Verification items for this drawing (mm, ordinates from the low corner). Round coordinates to 2 decimals unless told otherwise and drop trailing zeros. Loops run counter-clockwise (first coordinate to the right, second up) from the corner with the lowest first, then second, coordinate; pieces in that order, holes last. Notation, with made-up numbers: (-11, -9) - (25, -9) arc R7 cw to (25, 4) - close; hole circle Ø6 at (85.25, 76.25). An arc over 180 degrees is marked (long way). Answer in a Markdown table with one row per item. Add a question column.
(1) Cross-section at B-B on z = 360. Enter the section's corners in (x, y) (1 decimal).
(2) Thickness scan on line 1 along X through (y, z) = (10.25, 397); line 2 along X through (y, z) = (4.25, 385.5). Record the ranges inside material, lowest first.
(3) Gauge pin test, flat end, axial feed: pin 1 (5 mm diameter, centred on x = 221.5, y = 13.5, fed in from -Z) (1 decimal). Record the tip position at first contact, or that the pin passes through.
(4) Cross-section at A-A on y = 12.75. Enter the section's corners in (x, z) (1 decimal), then the cut area to 3 significant figures.
(5) Cross-section at C-C on z = 103.5. Enter the section's corners in (x, y) (1 decimal), then the cut area to 3 significant figures.
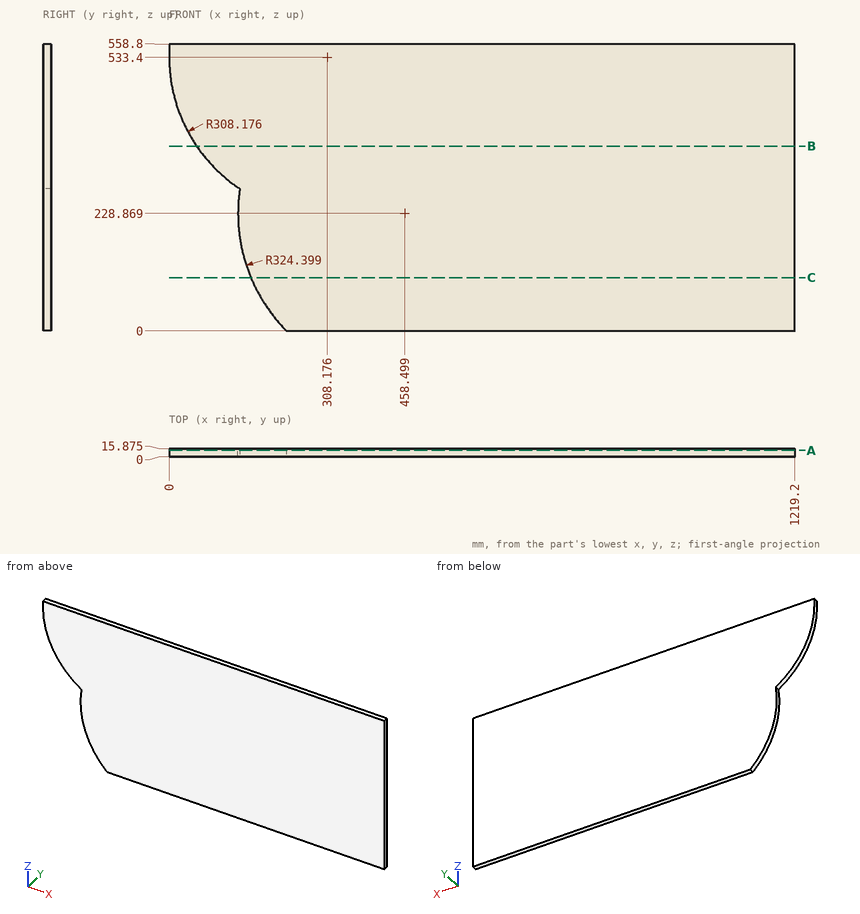
Answers:
| question | item | result |
|---|---|---|
| 1 | outline | (53.4, 0) - (1219.2, 0) - (1219.2, 15.9) - (53.4, 15.9) - close |
| 2 | line 1 | x = 31.83 to 1219.2 |
| 2 | line 2 | x = 37.81 to 1219.2 |
| 3 | pin 1 | stops at z = 4.7 |
| 4 | outline | (0, 533.4) arc R308.2 ccw to (137.6, 276.7) arc R324.4 ccw to (228.6, 0) - (1219.2, 0) - (1219.2, 558.8) - (0, 558.8) - close |
| 4 | area | 627,000 mm^2 |
| 5 | outline | (159.3, 0) - (1219.2, 0) - (1219.2, 15.9) - (159.3, 15.9) - close |
| 5 | area | 16,800 mm^2 |
